Build history of the part. All positions in model axes, mm. A direction names the side the tool comes from. Coordinates: 2 decimals unless noted, no trailing zeros. Loops run counter-clockwise (first coordinate to the right, second up) from the corner with the lowest first, then second, coordinate; pieces in that order, holes last.
Item 1: Cut at B-B (z = 0). List the corners of the cut face in (x, y), and give its area (3 significant figures).
Item 2: Cut at A-A (x = 0). List the corners of the cut face in (y, z), and give its area (3 significant figures).
Item 3: Cut at C-C (y = 7.75). List the corners of the cut face in (x, z), and give its area (3 significant figures).
Item 4: Drill centre lines: line 1 along Z through (x, y) = (0, 21); line 2 along X through (y, z) = (10.25, 0). Where is each one in solid material? Low to high.
Item 5: Flat gauge pins, fed straight in: pin 1 (1 mm diameter, centred on y = 6, z = 1.5, fed in from -X); pin 2 (3 mm diameter, centred on x = -2, y = 3.5, fed in from -Z); pin 3 (4 mm diameter, centred on y = 8, z = -1.5, fed in from -X). Where does each tip first touch, or does it go through?
Item 6: Mould opens along Z. For faces 3 (the face through (2.44, 20.63, -0.54)), 4 (the face through (0, 11.5, 3.5)), 5 (the face through (-1.3, 12, 2.4)), 6 (the face through (-0.07, 15.18, -1.5)) say: released by +Z, released by -Z, zero draft, split by the parting line, or undercut.
Item 7: 3-axis set-ups, long thin cutter, end or side, ignore diameter. For faces 1 (the face through (2.75, 11.5, 0)), 2 (the face through (2, 6, 0)): which of +Z, -Z, +X, -X, +Y, -Y reach the whole face in a straight line?
Item 8: Cut at D-D (y = 25.25). List the corners of the cut face in (x, z), and give its area (3 significant figures).
from build123d import *

# Parameters (mm, degrees)
CUT_EXTRUDE1_REACH = 32.406


with BuildPart() as part:
    # Sketch1 → Revolve1 (revolve)
    with BuildSketch(Plane(origin=(0, 0, 0), x_dir=(0, 0, -1), z_dir=(1, 0, 0))):
        Polygon((-1.5, 0.2), (-1.5, 29.75), (-1.75, 30), (-2, 30), (-2.5, 29.5), (-2.5, 12), (-3.5, 12), (-3.5, 11), (-2, 11), (-2, 0.2), (-1.8, 0), (-1.7, 0), align=None)
    revolve(axis=Axis((0, 30, 0), (0, -1, 0)))

    # Sketch2 → Cut-Extrude1 (cut, up to next)
    with BuildSketch(Plane(origin=(0, 0, 0), x_dir=(1, 0, 0), z_dir=(0, 1, 0)), mode=Mode.PRIVATE) as cut_extrude1_sk1:
        with BuildLine():
            Line((-2.75, 2.165063509), (-2.75, -2.165063509))
            ThreePointArc((-2.75, -2.165063509), (-3.5, 0), (-2.75, 2.165063509))
        make_face()
    cut_extrude1_tool1 = extrude(cut_extrude1_sk1.sketch, amount=CUT_EXTRUDE1_REACH, mode=Mode.PRIVATE) & part.part
    # Sketch2 → Cut-Extrude1 (cut, up to next)
    with BuildSketch(Plane(origin=(0, 0, 0), x_dir=(1, 0, 0), z_dir=(0, 1, 0)), mode=Mode.PRIVATE) as cut_extrude1_sk2:
        with BuildLine():
            Line((2.75, 2.165063509), (2.75, -2.165063509))
            ThreePointArc((2.75, -2.165063509), (3.5, 0), (2.75, 2.165063509))
        make_face()
    cut_extrude1_tool2 = extrude(cut_extrude1_sk2.sketch, amount=CUT_EXTRUDE1_REACH, mode=Mode.PRIVATE) & part.part
    add(cut_extrude1_tool1.solids().sort_by_distance((-3.052938, 0, 0))[0], mode=Mode.SUBTRACT)
    add(cut_extrude1_tool2.solids().sort_by_distance((3.052938, 0, 0))[0], mode=Mode.SUBTRACT)


solid = part.part
Filled sheet:
1. outline: (-2.75, 11) - (-2, 11) - (-2, 0.2) - (-1.8, 0) - (-1.7, 0) - (-1.5, 0.2) - (-1.5, 29.75) - (-1.75, 30) - (-2, 30) - (-2.5, 29.5) - (-2.5, 12) - (-2.75, 12) - close; (1.5, 0.2) - (1.7, 0) - (1.8, 0) - (2, 0.2) - (2, 11) - (2.75, 11) - (2.75, 12) - (2.5, 12) - (2.5, 29.5) - (2, 30) - (1.75, 30) - (1.5, 29.75) - close
1. area: 49.1 mm2
2. outline: (0, -1.8) - (0.2, -2) - (11, -2) - (11, -3.5) - (12, -3.5) - (12, -2.5) - (29.5, -2.5) - (30, -2) - (30, -1.75) - (29.75, -1.5) - (0.2, -1.5) - (0, -1.7) - close; (0, 1.7) - (0.2, 1.5) - (29.75, 1.5) - (30, 1.75) - (30, 2) - (29.5, 2.5) - (12, 2.5) - (12, 3.5) - (11, 3.5) - (11, 2) - (0.2, 2) - (0, 1.8) - close
2. area: 50.6 mm2
3. outline: circle Ø4 at (0, 0); hole circle Ø3 at (0, 0)
3. area: 5.50 mm2
4. line 1: z = -2.5 to -1.5, 1.5 to 2.5
4. line 2: x = -2 to -1.5, 1.5 to 2
5. pin 1: stops at x = -1.73
5. pin 2: stops at z = -1.94
5. pin 3: stops at x = -2
6. face 3: split by the parting line
6. face 4: released by +Z
6. face 5: zero draft
6. face 6: undercut
7. face 1: +Z, -Z, +X, +Y, -Y
7. face 2: -Y
8. outline: circle Ø5 at (0, 0); hole circle Ø3 at (0, 0)
8. area: 12.6 mm2
